```python
from build123d import *

# Parameters (mm, degrees)
EXTRUDE_1_DEPTH = 6
SKETCH_2_R      = 2
EXTRUDE_2_DEPTH = 6
SKETCH_6_R      = 1.5
EXTRUDE_3_DEPTH = 8


with BuildPart() as part:
    # 草图1 → 拉伸1 (new body)
    with BuildSketch(Plane.XY):
        Polygon((1.58771324, -2.75), (3.175426481, 0), (1.58771324, 2.75), (-1.58771324, 2.75), (-3.175426481, 0), (-1.58771324, -2.75), align=None)
    extrude(amount=EXTRUDE_1_DEPTH)

    # 草图2 → 拉伸2 (add)
    with BuildSketch(Plane.XY.offset(6)):
        Circle(SKETCH_2_R)
    extrude(amount=EXTRUDE_2_DEPTH)

    # 草图6 → 拉伸3 (add)
    with BuildSketch(Plane(origin=(0, 0, 0), x_dir=(-1, 0, 0), z_dir=(0, 0, -1))):
        with Locations(Location((0, 0, 0), (0, 0, 180))):
            Circle(SKETCH_6_R)
    extrude(amount=EXTRUDE_3_DEPTH)


solid = part.part
```
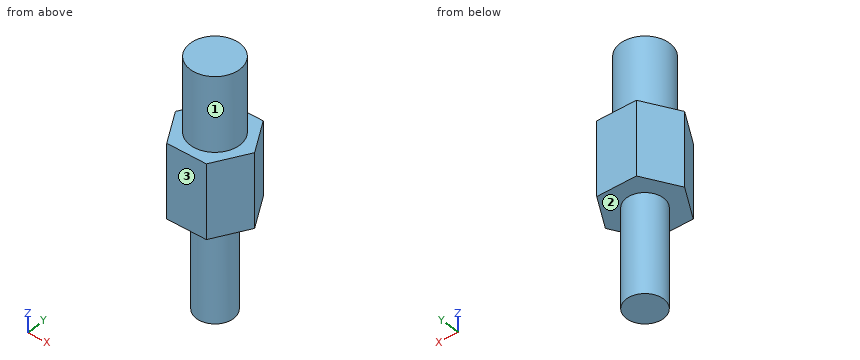
Input: part model. Units: mm. Frame: model coordinates. Face numbers are marked on the shaded views. A direction names the side the tool comes from. Coordinates: 2 decimals unless noted, no trailing zeros. Loops run counter-clockwise (first coordinate to the right, second up) from the corner with the lowest first, then second, coordinate; pieces in that order, holes last. Notation, with made-up numbers: M -16.5,79.25 L 21.5,79.25 A20 ccw 21.5,104.25 Z; hole C -1,63 d8. An arc over 180 degrees is marked long. Use a Markdown table: item, result. Add a question column.
1) Line query: L1, parallel to Z at x = 2, y = 1.3; L2, parallel to Z at x = -1.75, y = 0.5; L3, parallel to X at y = -0.55, z = 2.5. Output: solid intervals per line, ascending. Write a range as from..to.
2) Section A-A, the plane x = 0. Return the cut outline in (y, z).
3) Pin query (flat end, axial travel): P1, Ø1, axis at x = 0, z = -3, coming from the +Y side. Return the tip coordinate at first contact, or that it passes through.
4) Section C-C, the plane z = 3.25. Return the cut outline in (x, y), plus the area to 3 significant figures.
5) Section B-B, the plane y = -0.85. Return the cut outline in (x, z), plus the area to 3 significant figures.
6) Section D-D, the plane y = -1.7. Return the cut outline in (x, z), plus the area to 3 significant figures.
7) Set-up query: the marked faces 1, 2 and 3. Return all of +Z, -Z, +X, -X, +Y, -Y with unobstructed straight access to the full face (end or side cutting, diameter ignored); none if empty.
Answer below:
| question | item | result |
|---|---|---|
| 1 | L1 | 0..6 |
| 1 | L2 | 0..12 |
| 1 | L3 | -2.86..2.86 |
| 2 | outline | M -2.75,0 L -1.5,0 L -1.5,-8 L 1.5,-8 L 1.5,0 L 2.75,0 L 2.75,6 L 2,6 L 2,12 L -2,12 L -2,6 L -2.75,6 Z |
| 3 | P1 | y = 1.5 |
| 4 | outline | M -3.18,0 L -1.59,-2.75 L 1.59,-2.75 L 3.18,0 L 1.59,2.75 L -1.59,2.75 Z |
| 4 | area | 26.2 mm2 |
| 5 | outline | M -2.68,0 L -1.24,0 L -1.24,-8 L 1.24,-8 L 1.24,0 L 2.68,0 L 2.68,6 L 1.81,6 L 1.81,12 L -1.81,12 L -1.81,6 L -2.68,6 Z |
| 5 | area | 73.7 mm2 |
| 6 | outline | M -2.19,0 L 2.19,0 L 2.19,6 L 1.05,6 L 1.05,12 L -1.05,12 L -1.05,6 L -2.19,6 Z |
| 6 | area | 39.0 mm2 |
| 7 | face 1 | +Z |
| 7 | face 2 | -Z |
| 7 | face 3 | +Z, -Z, +X, -X, -Y |
